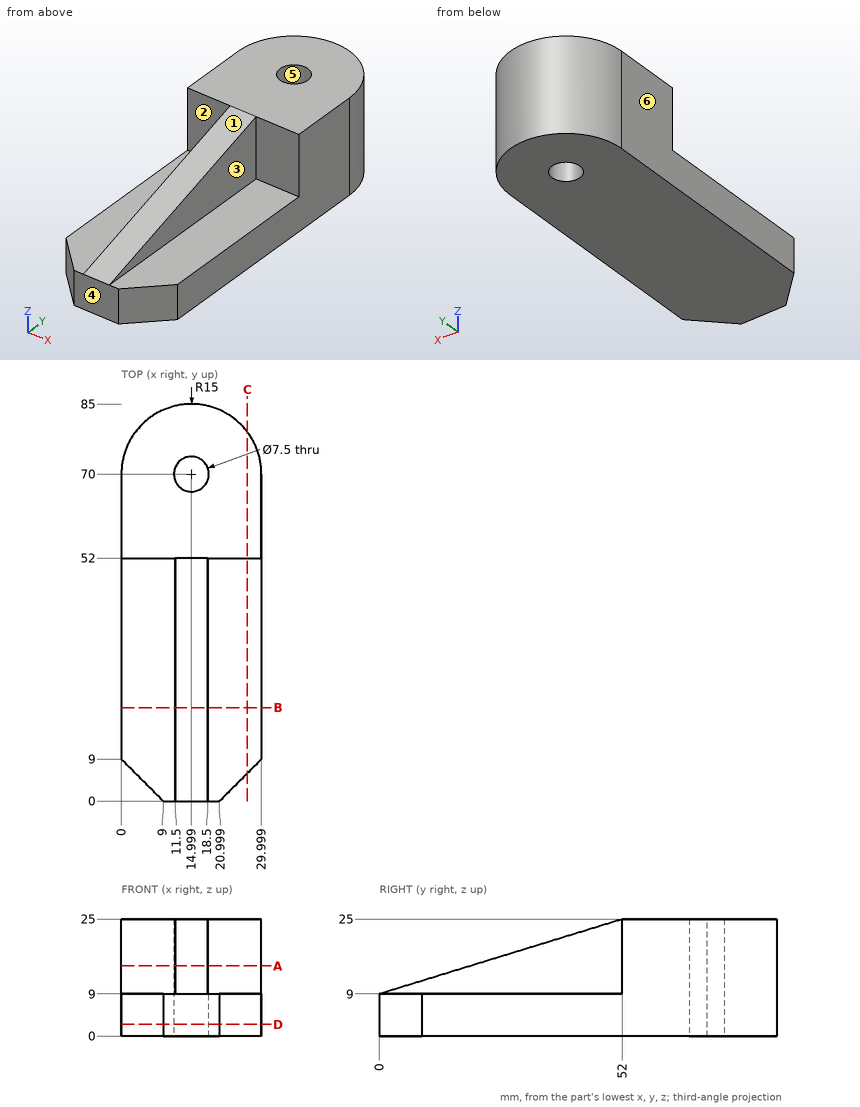
Check sheet for the drawn part. Datum: minimum x, y, z corner. Units: mm. A direction names the side the tool comes from. Give positions to 0.01 mm unless a question says otherwise; leave off trailing zeros. Order: outer loops, then holes, each group sorted by start corner. A loop starts at its lowest first (then second) coordinate and runs counter-clockwise, first axis right, second up. Notation, with made-up numbers: (-22.75, 68) - (-8.75, 68) arc R18 cw to (-8.75, 101) - close; hole circle Ø4 at (13, 41). An arc over 180 degrees is marked (long way). Answer as a JSON object with one key per item and string values.
(1) Cross-section at C-C (x = 27). Record the cut outline in (y, z), then the cut area to 3 significant figures.
Report:
{"outline": "(6, 0) - (79, 0) - (79, 25) - (52, 25) - (52, 9) - (6, 9) - close", "area": "1,090 mm^2"}
(2) Cross-section at D-D (z = 2.5). Record the cut outline in (x, y).
Report:
{"outline": "(0, 9) - (9, 0) - (21, 0) - (30, 9) - (30, 70) arc R15 ccw to (0, 70.12) - close; hole circle Ø7.5 at (15, 70)"}
(3) Cross-section at A-A (z = 15). Record the cut outline in (x, y).
Report:
{"outline": "(0, 52) - (11.5, 52) - (11.5, 19.5) - (18.5, 19.5) - (18.5, 52) - (30, 52) - (30, 70) arc R15 ccw to (0, 70.12) - close; hole circle Ø7.5 at (15, 70)"}
(4) Draft check along Y on the marked faces 4, 5 and 6. Enter one of: released by +Y, released by -Y, zero draft, split by the parting line, or undercut.
Report:
{"face 4": "released by -Y", "face 5": "undercut", "face 6": "zero draft"}
(5) Material ranges on line 1 (Z direction, x = 22.25, y = 41.5); line 2 (X direction, y = 69.5, z = 16) (1 decimal); line 3 (X direction, y = 69, z = 15.5) (1 decimal), recorded low to high.
Report:
{"line 1": "0 to 9", "line 2": "0 to 11.3, 18.7 to 30", "line 3": "0 to 11.4, 18.6 to 30"}
(6) Cross-section at B-B (y = 20). Record the cut outline in (x, z).
Report:
{"outline": "(0, 0) - (30, 0) - (30, 9) - (18.5, 9) - (18.5, 15.15) - (11.5, 15.15) - (11.5, 9) - (0, 9) - close"}
(7) Depth check by flat-ended pin: pin 1 Ø1 at (x, z) = (8.5, 13) entering from -Y; pin 2 Ø8 at (x, z) = (20, 13.5) entering from +Y; pin 3 Ø12.5 at (x, y) = (5, 26) entering from +Z. Enter the tip coordinate at first touch or a pass-through.
Report:
{"pin 1": "y = 52", "pin 2": "y = 84.97", "pin 3": "z = 9"}
(8) Tool access check on the marked faces 1, 2 and 3. Record the directions out of +Z, -Z, +X, -X, +Y, -Y that give a thin tool (end or side, any length) a straight path to the whole face; none if there is none.
Report:
{"face 1": "+Z, +X, -X, -Y", "face 2": "+Z, -X, -Y", "face 3": "+Z, +X, -Y"}
